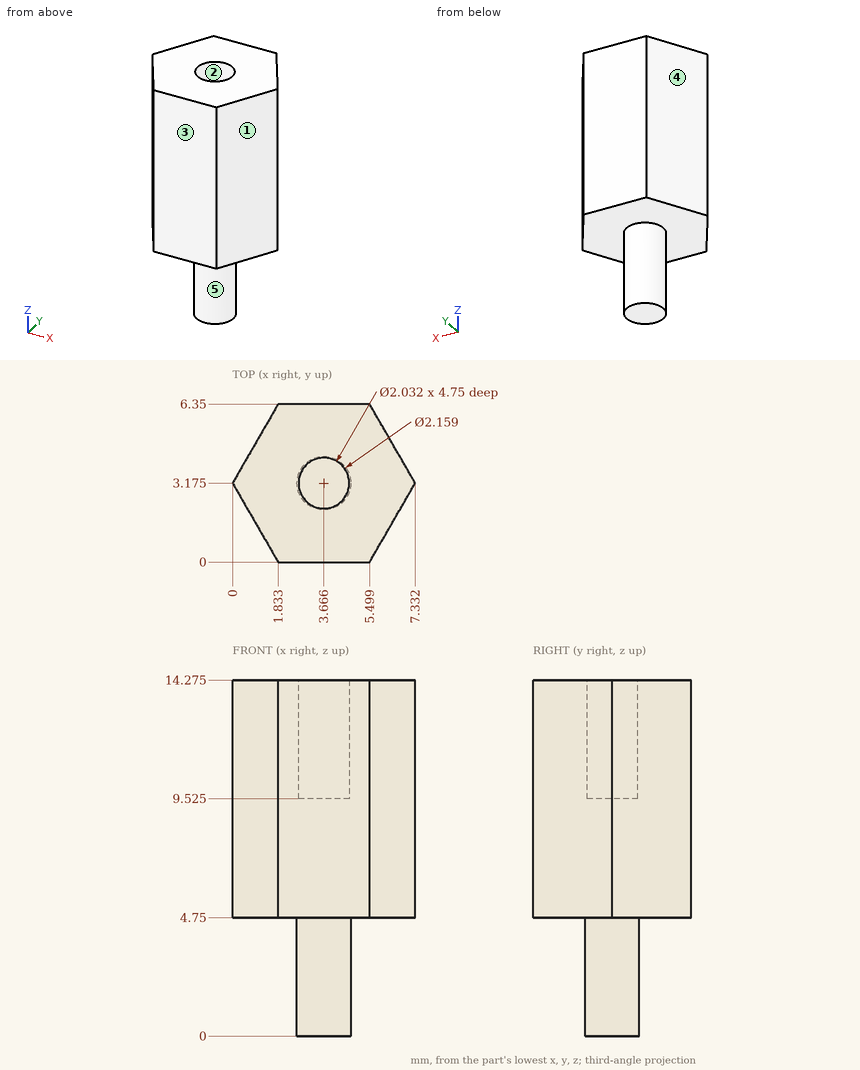
Geometry check sheet. Reference: drawing and pictorial views, mm from the part's lowest x, y, z. A direction names the side the tool comes from. Give positions to 0.01 mm unless a question says otherwise; leave off trailing zeros.
1. Mould release check, pull along X, two halves, no side actions. Record for the marked faces 1, 2 and 3: released by +X, released by -X, zero draft, split by the parting line, or undercut.
2. Thickness scan on line 1 (X direction, y = 3.75, z = 12.75) (1 decimal); line 2 (X direction, y = 0.5, z = 7.5) (1 decimal); line 3 (Y direction, x = 6.75, z = 7.75) (1 decimal). Record the ranges inside material, lowest first.
3. Go/stop test with flat-tipped pins: pin 1 Ø3 at (y, z) = (2, 11.5) entering from +X; pin 2 Ø2 at (y, z) = (1, 4) entering from -X (1 decimal); pin 3 Ø1 at (x, y) = (4.5, 5.5) entering from -Z. Record where each tip stops, or that it passes through.
4. Set-up check for the marked faces 4 and 5: record each of +Z, -Z, +X, -X, +Y, -Y from which the full face is reachable in a straight line by a thin tool's end or side.
Geometry says:
1. face 1: released by +X
1. face 2: undercut
1. face 3: zero draft
2. line 1: x = 0.3 to 2.8, 4.5 to 7
2. line 2: x = 1.5 to 5.8
2. line 3: y = 2.2 to 4.2
3. pin 1: stops at x = 7.33
3. pin 2: stops at x = 0.9
3. pin 3: stops at z = 4.75
4. face 4: +Z, -Z, -X, +Y
4. face 5: -Z
